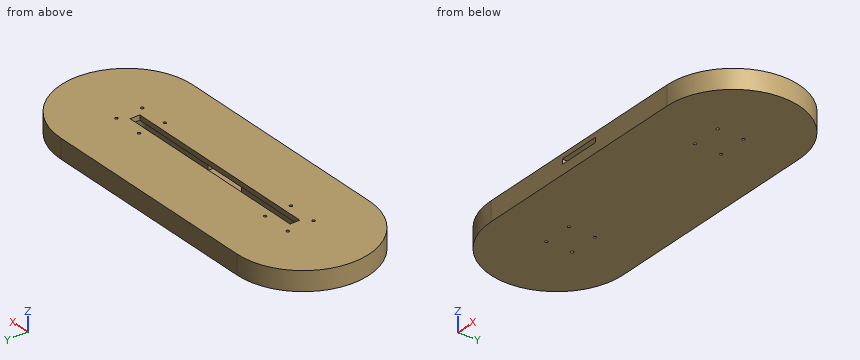
from build123d import *

# Parameters (mm, degrees)
PAD_DEPTH       = 9
POCKET_DEPTH    = 6
SKETCH002_W     = 26.5
SKETCH002_H     = 35
POCKET001_DEPTH = 6
SKETCH003_W     = 127
SKETCH003_H     = 5.95
PAD001_DEPTH    = 3
SKETCH004_R     = 0.85
POCKET002_DEPTH = 485.929265
SKETCH005_W     = 26.5
SKETCH005_H     = 7.75
PAD002_DEPTH    = 3


with BuildPart() as part:
    # Sketch → Pad (new body)
    with BuildSketch(Plane.XY):
        with BuildLine():
            ThreePointArc((-70, 41), (-111, 0), (-70, -41))
            Line((-70, -41), (70, -41))
            ThreePointArc((70, -41), (111, 0), (70, 41))
            Line((-70, 41), (70, 41))
        make_face()
    extrude(amount=PAD_DEPTH)

    # Sketch001 (on Face6 of Pad) → Pocket (cut)
    with BuildSketch(Plane.XY.offset(9)):
        with BuildLine():
            ThreePointArc((-62.5, 6), (-68.5, 0), (-62.5, -6))
            Line((-62.5, -6), (62.5, -6))
            ThreePointArc((62.5, -6), (68.5, 0), (62.5, 6))
            Line((-62.5, 6), (62.5, 6))
        make_face()
    extrude(amount=-POCKET_DEPTH, mode=Mode.SUBTRACT)

    # Sketch002 (on Face5 of Pocket) → Pocket001 (cut)
    with BuildSketch(Plane.XY.offset(9)):
        with Locations((0, -23.5)):
            Rectangle(SKETCH002_W, SKETCH002_H)
    extrude(amount=-POCKET001_DEPTH, mode=Mode.SUBTRACT)

    # Sketch003 (on Face5 of Pocket001) → Pad001 (join)
    with BuildSketch(Plane.XY.offset(9)):
        with BuildLine():
            ThreePointArc((-70, 41), (-111, 0), (-70, -41))
            Line((-70, -41), (70, -41))
            ThreePointArc((70, -41), (111, 0), (70, 41))
            Line((-70, 41), (70, 41))
        make_face()
        Rectangle(SKETCH003_W, SKETCH003_H, mode=Mode.SUBTRACT)
    extrude(amount=PAD001_DEPTH)

    # Sketch004 (on Face12 of Pad001) → Pocket002 (cut, through all)
    with BuildSketch(Plane.XY.offset(12)):
        with Locations((-68, -8)):
            Circle(SKETCH004_R)
        with Locations((-50, -8)):
            Circle(SKETCH004_R)
        with Locations((-50, 8)):
            Circle(SKETCH004_R)
        with Locations((-68, 8)):
            Circle(SKETCH004_R)
    pocket002 = extrude(amount=-POCKET002_DEPTH, mode=Mode.SUBTRACT)

    # Sketch005 (on Face10 of Pocket002) → Pad002 (join)
    with BuildSketch(Plane.XY.offset(3)):
        with Locations((0, -37.125)):
            Rectangle(SKETCH005_W, SKETCH005_H)
    extrude(amount=PAD002_DEPTH)

    # Mirrored: Pocket002 across Sketch004 V_Axis
    add(pocket002.mirror(Plane(origin=(0, 0, 12), x_dir=(0, 0, 1), z_dir=(1, 0, 0))), mode=Mode.SUBTRACT)


solid = part.part
The listing builds one solid part. Answer for the finished solid, in the listing's coordinates (mm). Coordinates: 2 decimals unless noted, no trailing zeros. Write each loop counter-clockwise with the first axis right and the second up, starting at its lowest first coordinate (ties: lowest second). Pieces come first, ordered by that corner, then holes. Notation, with made-up numbers: M -10.75,57.25 L 8.25,57.25 A21 cw 8.25,61.25 Z; hole C 22,36.5 d2. An arc over 180 degrees is marked long. Write each question's results on one line, items separated by ' | '.
Item 1: Consider probe 1 along Y at (x, z) = (-50, 8.5); probe 2 along Y at (x, z) = (56, 4.75); probe 3 along Y at (x, z) = (22.5, 10.5) (3 decimals). Determine where each line is inside the solid, lowest interval first. Write a range as [from, to].
Answer below:
probe 1: [-41, -8.85], [-7.15, -6], [6, 7.15], [8.85, 41] | probe 2: [-41, -6], [6, 41] | probe 3: [-41, -2.975], [2.975, 41]
Item 2: The part is cut by section A-A on y = 0. Determine the outline of the cut face in (x, z).
Answer below:
outline: M -111,0 L 111,0 L 111,12 L 63.5,12 L 63.5,9 L 68.5,9 L 68.5,3 L -68.5,3 L -68.5,9 L -63.5,9 L -63.5,12 L -111,12 Z
Item 3: Given P1, Ø1.5, axis at y = -1.5, z = 11, coming from the -X side; P2, Ø4, axis at x = 82.5, z = 3.5, coming from the -Y side; P3, Ø1.8, axis at y = -15.5, z = 4.5, coming from the -X side, each flat-ended and moving along its own axis, determine where each tip first touches the part or whether it passes through.
Answer below:
P1: x = -110.99 | P2: y = -39.63 | P3: x = -108.31
Item 4: The part is cut by section C-C on y = -18. Determine the outline of the cut face in (x, z), and give its area (3 significant figures).
Answer below:
outline: M -106.84,0 L 106.84,0 L 106.84,12 L -106.84,12 Z; hole M -13.25,3 L 13.25,3 L 13.25,9 L -13.25,9 Z | area: 2,410 mm2
Item 5: The part is cut by section D-D on y = -28. Determine the outline of the cut face in (x, z), and give its area (3 significant figures).
Answer below:
outline: M -99.95,0 L 99.95,0 L 99.95,12 L -99.95,12 Z; hole M -13.25,3 L 13.25,3 L 13.25,9 L -13.25,9 Z | area: 2,240 mm2
Item 6: The part is cut by section B-B on x = -22. Determine the outline of the cut face in (y, z) (3 decimals).
Answer below:
outline: M -41,0 L 41,0 L 41,12 L 2.975,12 L 2.975,9 L 6,9 L 6,3 L -6,3 L -6,9 L -2.975,9 L -2.975,12 L -41,12 Z
